Source: CAD feature listing. Evaluate the final solid. Frame: model axes, mm. A direction names the side the tool comes from. Give positions to 0.01 mm unless a question says otherwise; leave off trailing zeros. Loops run counter-clockwise (first coordinate to the right, second up) from the corner with the lowest first, then second, coordinate; pieces in that order, holes last. Notation, with made-up numbers: (-35, 63) -> (-4, 63) arc R10 cw to (-4, 75) -> close; hole circle Ø3 at (64.5, 70). An arc over 180 degrees is marked (long way). Put each result on its own line as item: value.
```python
from build123d import *

# Parameters (mm, degrees)
ESBO_O1_W                = 38
ESBO_O1_H                = 80
ESBO_O1_R                = 1.5
ESBO_O1_W_2              = 8
ESBO_O1_H_2              = 24
ESBO_O1_W_3              = 28
ESBO_O1_H_3              = 40
RESSALTO_EXTRUS_O1_DEPTH = 5
CORTE_EXTRUS_O1_DEPTH    = 56.398555938
ESBO_O6_R                = 8.5
CORTE_EXTRUS_O3_DEPTH    = 62.919302322
ESBO_O6_3_R              = 11
ESBO_O6_3_R_2            = 8.5
CORTE_EXTRUS_O4_DEPTH    = 2
FURO_ROSCADO_DE_M41_D    = 4
FILETE1_R                = 16
FILETE2_R                = 5
FILETE3_R                = 8
ESBO_O9_R                = 1.6
CORTE_EXTRUS_O9_DEPTH    = 62.919302322


with BuildPart() as part:
    # Esbo_o1 → Ressalto-extrus_o1 (new body)
    # profile 1 of 2: a face of its own
    with BuildSketch(Plane.XY):
        Rectangle(ESBO_O1_W, ESBO_O1_H)
        with Locations((-15, 19.5)):
            Circle(ESBO_O1_R, mode=Mode.SUBTRACT)
        with Locations((-15, -19.5)):
            Circle(ESBO_O1_R, mode=Mode.SUBTRACT)
        with Locations((3, -19.5)):
            Circle(ESBO_O1_R, mode=Mode.SUBTRACT)
        with Locations((3, 19.5)):
            Circle(ESBO_O1_R, mode=Mode.SUBTRACT)
        with Locations((3, 30.5)):
            Circle(ESBO_O1_R, mode=Mode.SUBTRACT)
        with Locations((-15, 30.5)):
            Circle(ESBO_O1_R, mode=Mode.SUBTRACT)
        with Locations((3, -30.5)):
            Circle(ESBO_O1_R, mode=Mode.SUBTRACT)
        with Locations((-15, -30.5)):
            Circle(ESBO_O1_R, mode=Mode.SUBTRACT)
        with Locations((-6, 25)):
            Rectangle(ESBO_O1_W_2, ESBO_O1_H_2, mode=Mode.SUBTRACT)
        with Locations((-6, -25)):
            Rectangle(ESBO_O1_W_2, ESBO_O1_H_2, mode=Mode.SUBTRACT)
    # profile 2 of 2: a face of its own
    with BuildSketch(Plane.XY):
        with Locations((33, 0)):
            Rectangle(ESBO_O1_W_3, ESBO_O1_H_3)
    extrude(amount=RESSALTO_EXTRUS_O1_DEPTH)

    # Esbo_o2 → Corte-extrus_o1 (cut, through all)
    with BuildSketch(Plane(origin=(19, 0, 0), x_dir=(0, 0, -1), z_dir=(1, 0, 0))):
        Polygon((-2, 25), (0, 28.464101615), (0, 21.535898385), align=None)
        Polygon((-2, -25), (0, -21.535898385), (0, -28.464101615), align=None)
    extrude(amount=-CORTE_EXTRUS_O1_DEPTH, mode=Mode.SUBTRACT)

    # Esbo_o6 → Corte-extrus_o3 (cut, through all)
    with BuildSketch(Plane.XY.offset(5)):
        with Locations((32, 0)):
            Circle(ESBO_O6_R)
    extrude(amount=-CORTE_EXTRUS_O3_DEPTH, mode=Mode.SUBTRACT)

    # Esbo_o6_3 → Corte-extrus_o4 (cut)
    with BuildSketch(Plane.XY.offset(5)):
        with Locations((32, 0)):
            Circle(ESBO_O6_3_R)
        with Locations((32, 0)):
            Circle(ESBO_O6_3_R_2, mode=Mode.SUBTRACT)
    extrude(amount=-CORTE_EXTRUS_O4_DEPTH, mode=Mode.SUBTRACT)

    # Furo roscado de M41 (through all)
    with Locations(Plane(origin=(-8.290173831, 15.833247685, 5), x_dir=(1, 0, 0), z_dir=(0, 0, 1))):
        with Locations((40.290173831, -2.832747685), (40.290173831, -28.833747685)):
            Hole(FURO_ROSCADO_DE_M41_D / 2)

    # Filete1
    filete1_edges = [part.edges().sort_by_distance(p)[0] for p in [
        (47, 20, 2.5),
        (47, -20, 2.5),
    ]]
    fillet(filete1_edges, radius=FILETE1_R)

    # Filete2
    filete2_edges = [part.edges().sort_by_distance(p)[0] for p in [
        (19, -20, 2.5),
        (19, 20, 2.5),
    ]]
    fillet(filete2_edges, radius=FILETE2_R)

    # Filete3
    filete3_edges = [part.edges().sort_by_distance(p)[0] for p in [
        (19, -40, 2.5),
        (-19, -40, 2.5),
        (-19, 40, 2.5),
        (19, 40, 2.5),
    ]]
    fillet(filete3_edges, radius=FILETE3_R)

    # Esbo_o9 → Corte-extrus_o9 (cut, through all)
    with BuildSketch(Plane.XY):
        with Locations(Location((5, 0, 0), (0, 0, 180))):
            Circle(ESBO_O9_R)
        with Locations(Location((17, 0, 0), (0, 0, 180))):
            Circle(ESBO_O9_R)
    extrude(amount=CORTE_EXTRUS_O9_DEPTH, mode=Mode.SUBTRACT)


solid = part.part
```
(1) Line query: probe 1 along Y at (x, z) = (3, 2.9); probe 2 along Y at (x, z) = (-15, 2.7); probe 3 along Y at (x, z) = (5, 2.4). Output: solid intervals per line, ascending. Write a range as from..to.
Calculated:
probe 1: y = -40..-32, -29..-21, -18..18, 21..29, 32..40
probe 2: y = -38.93..-32, -29..-21, -18..18, 21..29, 32..38.93
probe 3: y = -40..-1.6, 1.6..40
(2) Section C-C on x = 17. Return loops of the section in (y, z).
Calculated:
outline: (-37.29, 0) -> (-28.46, 0) -> (-25, 2) -> (-21.54, 0) -> (-1.6, 0) -> (-1.6, 5) -> (-37.29, 5) -> close; (1.6, 0) -> (21.54, 0) -> (25, 2) -> (28.46, 0) -> (37.29, 0) -> (37.29, 5) -> (1.6, 5) -> close
(3) First-contact query: P1, Ø2.5, axis at y = 24.5, z = 3.5, coming from the +X side; P2, Ø1, axis at x = 29, z = 4, coming from the +Y side; P3, Ø2, axis at y = 23.5, z = 1.5, coming from the +X side. Flat tips, straight axial feed; report the tip coordinate or a pass-through.
Calculated:
P1: stops at x = 19.32
P2: stops at y = 20
P3: stops at x = 19.67
(4) Reachability of faces 1 (the flat face through (19, -29, 2)), 2 (the flat face through (-10, -25.2, 2.5)), 3 (the flat face through (27, 20, 2)), 4 (the flat face through (-14.437, 26.708, 1.014)) from +Z, -Z, +X, -X, +Y, -Y: full face, straight path, thin tool, end or side. Return the list, or none.
Calculated:
face 1: +Z, -Z, +X, -Y
face 2: +Z, -Z
face 3: +Z, -Z, +X, +Y
face 4: -Z, +X, -X
(5) Section A-A on y = -30.5. Return loops of the section in (x, z), then the cut area to 3 significant figures.
Calculated:
outline: (-19, 0) -> (-16.5, 0) -> (-16.5, 5) -> (-19, 5) -> close; (-13.5, 0) -> (-10, 0) -> (-10, 5) -> (-13.5, 5) -> close; (-2, 0) -> (1.5, 0) -> (1.5, 5) -> (-2, 5) -> close; (4.5, 0) -> (19, 0) -> (19, 5) -> (4.5, 5) -> close
area: 120 mm²
(6) Draft query along Y for faces 5 (the flat face through (-10, 24.8, 2.5)), 6 (the cylindrical face through (21, 21, 3)), 7 (the cylindrical face through (42.189, -15.437, 2.535)). Return one class per face: released by +Y, released by -Y, zero draft, split by the parting line, or undercut.
Calculated:
face 5: undercut
face 6: released by +Y
face 7: released by -Y
(7) Section B-B on x = 32. Give the number of separate pieces and of enclosed holes in the cut face, then the cut area to 3 significant figures.
Calculated:
separate pieces: 4
enclosed holes: 0
area: 64.7 mm²
